Verification items for the finished model (mm, model axes). Face numbers are marked on the shaded views. A direction names the side the tool comes from. Coordinates: 2 decimals unless noted, no trailing zeros. Order: outer loops, then holes, each group sorted by start corner. A loop starts at its lowest first (then second) coordinate and runs counter-clockwise, first axis right, second up. Notation, with made-up numbers: M 75.25,2 L 93.25,2 A22 cw 93.25,32 Z; hole C 22,-3.75 d6. An arc over 180 degrees is marked long. Return JSON: item names as keys, results as strings. Group by question number.
1. Section check A-A, the plane z = -12. Record the cut outline in (x, y).
2. Gauge pin test, flat ends, axial feed: pin 1 (7 mm diameter, centred on x = 10, z = 7.5, fed in from +Y); pin 2 (1 mm diameter, centred on y = 6, z = -13, fed in from +X). Record the tip position at first contact, or that the pin passes through.
3. Material ranges on line 1 along Z through (x, y) = (10, -2.3); line 2 along Y through (x, z) = (-0.6, -11); line 3 along Z through (x, y) = (12, -0.75), recorded low to high.
4. Mould release check, pull along Y, two halves, no side actions. Record for the marked faces 3, 4, 5 and 6: +Y half, -Y half, draft (parallel to the pull), parting line (faces both ways), or undercut.
5. Section check C-C, the plane y = 5. Record the cut outline in (x, z), plus the area to 3 significant figures.
6. Set-up check for the marked faces 1 and 2: record each of +Z, -Z, +X, -X, +Y, -Y from which the full face is reachable in a straight line by a thin tool's end or side.
7. Section check B-B, the plane x = 8.25. Record the cut outline in (y, z), plus the area to 3 significant figures.
8. Section check D-D, the plane x = 5. Record the cut outline in (y, z), plus the area to 3 significant figures.
```python
from build123d import *

# Parameters (mm, degrees)
EXTRUDE_1_DEPTH             = 16
HOLE_WIZARD_4_5_4_5_1_D     = 4.5
HOLE_WIZARD_4_5_4_5_1_DEPTH = 5
HOLE_WIZARD_4_5_4_5_1_TIP   = 1.351936393
HOLE_WIZARD_4_5_4_5_2_D     = 4.5
HOLE_WIZARD_4_5_4_5_2_DEPTH = 5
HOLE_WIZARD_4_5_4_5_2_TIP   = 1.351936393
CHAMFER_1_SIZE              = 0.5


with BuildPart() as part:
    # 草图6 → 拉伸-薄壁1 (new, symmetric)
    with BuildSketch(Plane.XY):
        Polygon((15, 0), (0, 0), (0, 7.5), (-3, 7.5), (-3, -3), (15, -3), align=None)
    extrude(amount=EXTRUDE_1_DEPTH, both=True)

    # Ø4.5 (4.5) 直径孔1
    with Locations(Plane(origin=(0, -1.729, -9.85), x_dir=(0, 0, 1), z_dir=(1, 0, 0))):
        with Locations((-1.15, -5.75), (20.85, -5.75)):
            Hole(HOLE_WIZARD_4_5_4_5_1_D / 2, depth=HOLE_WIZARD_4_5_4_5_1_DEPTH)
            with Locations((0, 0, -(HOLE_WIZARD_4_5_4_5_1_DEPTH + HOLE_WIZARD_4_5_4_5_1_TIP / 2))):  # 118° drill point
                Cone(0, HOLE_WIZARD_4_5_4_5_1_D / 2, HOLE_WIZARD_4_5_4_5_1_TIP, mode=Mode.SUBTRACT)

    # Ø4.5 (4.5) 直径孔2
    with Locations(Plane(origin=(0, 0, 0), x_dir=(1, 0, 0), z_dir=(0, 1, 0))):
        with Locations((10, -7.5), (10, 7.5)):
            Hole(HOLE_WIZARD_4_5_4_5_2_D / 2, depth=HOLE_WIZARD_4_5_4_5_2_DEPTH)
            with Locations((0, 0, -(HOLE_WIZARD_4_5_4_5_2_DEPTH + HOLE_WIZARD_4_5_4_5_2_TIP / 2))):  # 118° drill point
                Cone(0, HOLE_WIZARD_4_5_4_5_2_D / 2, HOLE_WIZARD_4_5_4_5_2_TIP, mode=Mode.SUBTRACT)

    # 倒角1
    chamfer_1_edges = [part.edges().sort_by_distance(p)[0] for p in [
        (-1.5, 7.5, 16),
        (-1.5, 7.5, -16),
        (15, -1.5, -16),
        (15, -1.5, 16),
    ]]
    chamfer(chamfer_1_edges, length=CHAMFER_1_SIZE)


solid = part.part
```
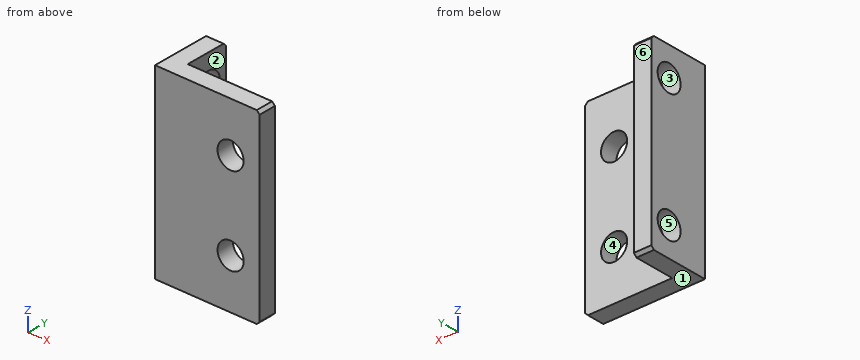
Answers follow:
{
 "1": {"outline": "M -3,-3 L 15,-3 L 15,0 L 0,0 L 0,2.01 L -3,2.01 Z; M -3,6.04 L 0,6.04 L 0,7.5 L -3,7.5 Z"},
 "2": {"pin 1": "y = 0", "pin 2": "x = 0"},
 "3": {"line 1": "-16 to -9.75, -5.25 to 5.25, 9.75 to 16", "line 2": "-3 to 1.77, 6.27 to 7.5", "line 3": "-16 to -8.53, -6.47 to 6.47, 8.53 to 16"},
 "4": {"face 3": "undercut", "face 4": "draft", "face 5": "undercut", "face 6": "+Y half"},
 "5": {"outline": "M -3,-16 L 0,-16 L 0,-13.03 L -3,-13.03 Z; M -3,-8.97 L 0,-8.97 L 0,8.97 L -3,8.97 Z; M -3,13.03 L 0,13.03 L 0,16 L -3,16 Z", "area": "71.7 mm^2"},
 "6": {"face 1": "-Z, +X, -X, +Y, -Y", "face 2": "+Z, -Z, +X, +Y"},
 "7": {"outline": "M -3,-16 L 0,-16 L 0,-8.91 L -3,-8.91 Z; M -3,-6.09 L 0,-6.09 L 0,6.09 L -3,6.09 Z; M -3,8.91 L 0,8.91 L 0,16 L -3,16 Z", "area": "79.0 mm^2"},
 "8": {"outline": "M -3,-16 L 0,-16 L 0,16 L -3,16 Z", "area": "96.0 mm^2"}
}
